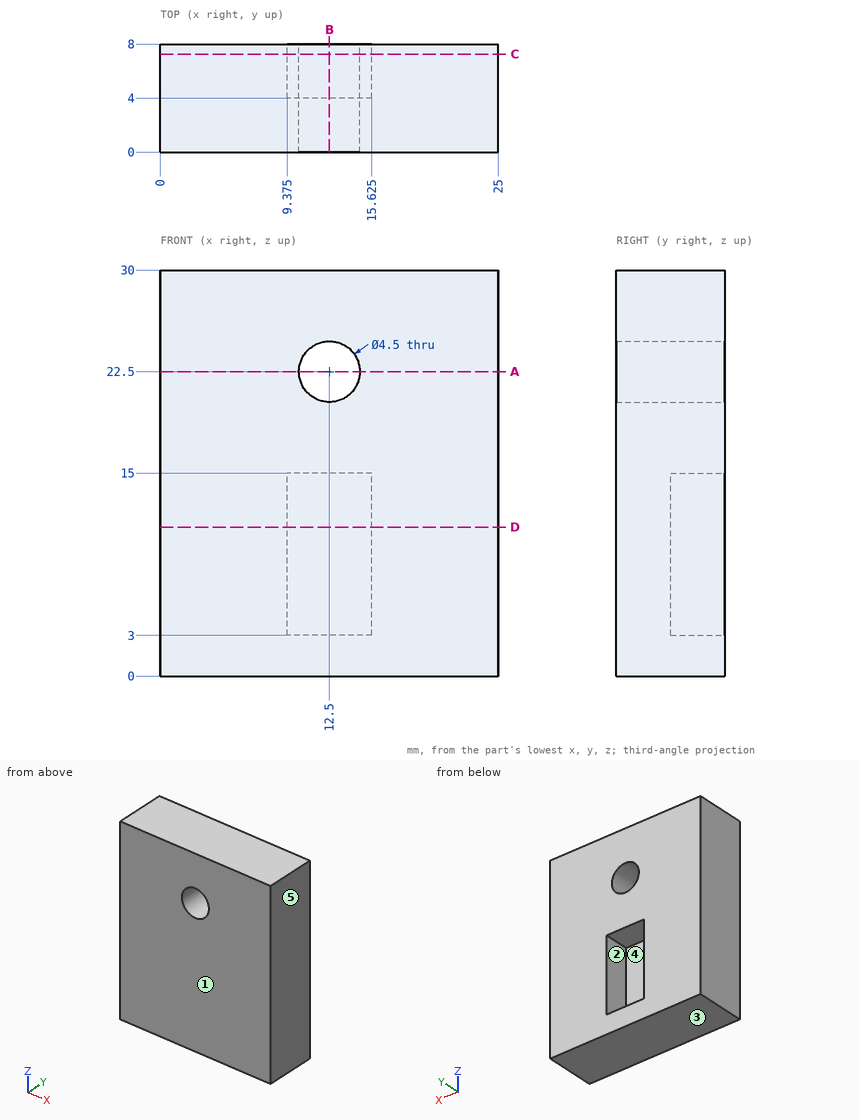
Can you work these out from the drawing? Everything is in mm from the part's minimum corner. A direction names the side the tool comes from. Coordinates: 2 decimals unless noted, no trailing zeros. Order: outer loops, then holes, each group sorted by start corner. A loop starts at its lowest first (then second) coordinate and runs counter-clockwise, first axis right, second up. Notation, with made-up numbers: M 73,-14 L 131,-14 A27 ccw 131,8 Z; hole C -13.75,59 d7. An arc over 180 degrees is marked long. Answer as CSV lines item,"result". Start each with the question number.
1. On a 3-axis mill with a long thin cutter (end or side, diameter ignored), from which of +Z, -Z, +X, -X, +Y, -Y can I reach the whole of each face in a straight line? I mean the marked faces 1 and 2. Say none if no direction works.
2. For pin 1 (2 mm diameter, centred on x = 18.5, y = 1, fed in from -Z); pin 2 (3.5 mm diameter, centred on x = 12.5, z = 22.5, fed in from -Y); pin 3 (5 mm diameter, centred on x = 12, z = 12, fed in from +Y), each with a flat end and sliding along its axis, tell me the tip position at first contact or that it passes through.
3. We'd pull the mould along X, two halves only. Please class the marked faces 3, 4 and 5: released by +X, released by -X, zero draft, split by the parting line, or undercut.
4. I need wall thicknesses on line 1 (Z direction, x = 12.5, y = 5.5); line 2 (X direction, y = 6.75, z = 22.5); line 3 (Z direction, x = 12.5, y = 2). Which ranges of each line are inside material? Lowest first, please. Write a range as [from, to].
5. I want a section at B-B, the plane x = 12.5. Write out the boundary of the cut face in (y, z), and give its area (3 significant figures).
6. I want a section at D-D, the plane z = 11. Write out the boundary of the cut face in (x, y) (3 decimals), and give its area (3 significant figures).
7. I want a section at C-C, the plane y = 7.25. Write out the boundary of the cut face in (x, z) (3 decimals).
8. I want a section at A-A, the plane z = 22.5. Write out the boundary of the cut face in (x, y).
Recorded:
1,face 1,"+Z, -Z, +X, -X, -Y"
1,face 2,"+Y"
2,pin 1,"stops at z = 0"
2,pin 2,"passes through"
2,pin 3,"stops at y = 4"
3,face 3,"zero draft"
3,face 4,"undercut"
3,face 5,"released by +X"
4,line 1,"z = [0, 3], [15, 20.25], [24.75, 30]"
4,line 2,"x = [0, 10.25], [14.75, 25]"
4,line 3,"z = [0, 20.25], [24.75, 30]"
5,outline,"M 0,0 L 8,0 L 8,3 L 4,3 L 4,15 L 8,15 L 8,20.25 L 0,20.25 Z; M 0,24.75 L 8,24.75 L 8,30 L 0,30 Z"
5,area,"156 mm2"
6,outline,"M 0,0 L 25,0 L 25,8 L 15.625,8 L 15.625,4 L 9.375,4 L 9.375,8 L 0,8 Z"
6,area,"175 mm2"
7,outline,"M 0,0 L 25,0 L 25,30 L 0,30 Z; hole M 9.375,3 L 15.625,3 L 15.625,15 L 9.375,15 Z; hole C 12.5,22.5 d4.5"
8,outline,"M 0,0 L 10.25,0 L 10.25,8 L 0,8 Z; M 14.75,0 L 25,0 L 25,8 L 14.75,8 Z"
